Geometry: final body of the model. Coordinates: model frame, mm. A direction names the side the tool comes from. Give positions to 0.01 mm unless a question says otherwise; leave off trailing zeros. Write each loop counter-clockwise with the first axis right and the second up, starting at its lowest first coordinate (ties: lowest second). Pieces come first, ordered by that corner, then holes. Notation, with made-up numbers: M 13.5,-16 L 25.5,-16 A30 cw 25.5,13 Z; hole C -1,-17 d8. An arc over 180 degrees is marked long. Use a Markdown table: item, result. Add a question column.
1) Section A-A on z = 0. Return the cut outline in (x, y) (3 decimals), then the cut area to 3 significant figures.
2) Set-up query: faces 4 (the flat face through (6, 4.989, 0)), 5 (the flat face through (-2, 8, 6)), 6 (the cylindrical face through (-5.77, 4.06, -0.25)). Return all of +Z, -Z, +X, -X, +Y, -Y with unobstructed straight access to the full face (end or side cutting, diameter ignored); none if empty.
3) Line query: line 1 (X direction, y = 8.75, z = 0); line 2 (Z direction, x = 0, y = 3) (3 decimals). Output: solid intervals per line, ascending.
4) Section C-C on y = 5.75. Return the cut outline in (x, z) (3 decimals).
5) Section D-D on y = 3.25. Return the cut outline in (x, z) (3 decimals), then the cut area to 3 significant figures.
6) Draft query along Z for faces 1 (the flat face through (-6, 0, -2)), 2 (the flat face through (5, 2, -4)), 3 (the cylindrical face through (-7.293, 4.437, -0.321)). Return one class per face: +Z half, -Z half, draft (parallel to the pull), parting line (faces both ways), or undercut.
7) Section B-B on x = 0. Return the cut outline in (y, z) (3 decimals).
8) Pin query (flat end, axial travel): pin 1 (2 mm diameter, centred on x = 5, y = 2, fed in from +Z); pin 2 (1.6 mm diameter, centred on x = 5.5, y = 3.5, fed in from -Z); pin 3 (3.5 mm diameter, centred on x = 6, z = -1.5, fed in from -Y). Return the tip coordinate at first contact, or that it passes through.
```python
from build123d import *

# Parameters (mm, degrees)
SKETCH1_R           = 7.3
BOSS_EXTRUDE1_DEPTH = 9
SKETCH2_R           = 6.9
CUT_EXTRUDE1_DEPTH  = 1
SKETCH3_R           = 5
CUT_EXTRUDE2_DEPTH  = 7
SKETCH4_R           = 5.775
CUT_EXTRUDE3_DEPTH  = 9
SKETCH5_W           = 4
SKETCH5_H           = 4.989216575
CUT_EXTRUDE4_DEPTH  = 6


with BuildPart() as part:
    # Sketch1 → Boss-Extrude1 (new body)
    with BuildSketch(Plane(origin=(0, 0, 0), x_dir=(1, 0, 0), z_dir=(0, 1, 0))):
        Circle(SKETCH1_R)
    extrude(amount=BOSS_EXTRUDE1_DEPTH)

    # Sketch2 → Cut-Extrude1 (cut)
    with BuildSketch(Plane(origin=(0, 9, 0), x_dir=(1, 0, 0), z_dir=(0, 1, 0))):
        Circle(SKETCH2_R)
    extrude(amount=-CUT_EXTRUDE1_DEPTH, mode=Mode.SUBTRACT)

    # Sketch3 → Cut-Extrude2 (cut)
    with BuildSketch(Plane.XZ):
        Circle(SKETCH3_R)
    extrude(amount=-CUT_EXTRUDE2_DEPTH, mode=Mode.SUBTRACT)

    # Sketch4 → Cut-Extrude3 (cut, through all)
    with BuildSketch(Plane(origin=(0, 8, 0), x_dir=(1, 0, 0), z_dir=(0, 1, 0))):
        Circle(SKETCH4_R)
    extrude(amount=-CUT_EXTRUDE3_DEPTH, mode=Mode.SUBTRACT)

    # Sketch5 → Cut-Extrude4 (cut)
    with BuildSketch(Plane(origin=(7.3, 0, 0), x_dir=(0, 0, -1), z_dir=(1, 0, 0))):
        with Locations((-2, 2.494608288)):
            Rectangle(SKETCH5_W, SKETCH5_H)
        with Locations((2, 2.494608288)):
            Rectangle(SKETCH5_W, SKETCH5_H)
    extrude(amount=-CUT_EXTRUDE4_DEPTH, mode=Mode.SUBTRACT)


solid = part.part
```
Found:
| question | item | result |
|---|---|---|
| 1 | outline | M -7.3,0 L -5.775,0 L -5.775,8 L -6.9,8 L -6.9,9 L -7.3,9 Z; M 5.775,4.989 L 7.3,4.989 L 7.3,9 L 6.9,9 L 6.9,8 L 5.775,8 Z |
| 1 | area | 17.6 mm² |
| 2 | face 4 | +X, -Y |
| 2 | face 5 | +Y |
| 2 | face 6 | +Y, -Y |
| 3 | line 1 | -7.3 to -6.9, 6.9 to 7.3 |
| 3 | line 2 | -7.3 to -5.775, 5.775 to 7.3 |
| 4 | outline | C 0,0 d14.6; hole C 0,0 d11.55 |
| 5 | outline | M 4.165,-4 A5.775 cw long 4.165,4 L 6.107,4 A7.3 ccw long 6.107,-4 Z |
| 5 | area | 49.5 mm² |
| 6 | face 1 | draft |
| 6 | face 2 | undercut |
| 6 | face 3 | parting line |
| 7 | outline | M 0,-7.3 L 9,-7.3 L 9,-6.9 L 8,-6.9 L 8,-5.775 L 0,-5.775 Z; M 0,5.775 L 8,5.775 L 8,6.9 L 9,6.9 L 9,7.3 L 0,7.3 Z |
| 8 | pin 1 | z = 6.11 |
| 8 | pin 2 | z = -5.59 |
| 8 | pin 3 | y = 4.99 |
